CAD build for the part. Positions are in the model's coordinates, mm. A direction names the side the tool comes from. Round coordinates to 2 decimals unless told otherwise and drop trailing zeros. Write each loop counter-clockwise with the first axis right and the second up, starting at its lowest first coordinate (ties: lowest second). Pieces come first, ordered by that corner, then holes. Notation, with made-up numbers: (-15.75, -30) - (37.25, -30) arc R33 cw to (37.25, -2) - close; hole circle Ø6 at (84.5, 77). An arc over 180 degrees is marked (long way). Answer in a Markdown table with one row per item.
```python
from build123d import *

# Parameters (mm, degrees)
F4_DEPTH  = 25.4
F5_DEPTH  = 50.8
F0_R      = 25.4
F0_R_2    = 12.7
F6_DEPTH  = 76.2
F7_DEPTH  = 76.2
F1_W      = 12.7
F1_H      = 34.925
F8_DEPTH  = 25.4
F9_W      = 12.7
F9_H      = 15.875
F10_DEPTH = 25.4


with BuildPart() as f4:
    # F2 (on Front) → F4 (new body, symmetric)
    with BuildSketch(Plane.XZ):
        Polygon((0, 50.8), (0, 0), (38.1, 0), align=None)
    extrude(amount=F4_DEPTH, both=True)

    # F3 (on Right) → F5 (cut)
    with BuildSketch(Plane.YZ):
        with BuildLine():
            ThreePointArc((-25.4, 0), (-21.997045, 12.7), (-12.7, 21.997045))
            Line((-12.7, 21.997045), (-12.7, 38.1))
            Line((-12.7, 38.1), (12.7, 38.1))
            Line((12.7, 38.1), (12.7, 50.8))
            Line((12.7, 50.8), (-25.4, 50.8))
            Line((-25.4, 50.8), (-25.4, 0))
        make_face()
    extrude(amount=F5_DEPTH, mode=Mode.SUBTRACT)

    # F0 (on Right) → F6 (join)
    with BuildSketch(Plane.YZ):
        Circle(F0_R)
        Circle(F0_R_2, mode=Mode.SUBTRACT)
    extrude(amount=F6_DEPTH)

    # F0 (on Right) → F7 (cut)
    with BuildSketch(Plane.YZ):
        Circle(F0_R_2)
    extrude(amount=F7_DEPTH, mode=Mode.SUBTRACT)

    # F1 (on Front) → F8 (cut, symmetric)
    with BuildSketch(Plane.XZ):
        with Locations((57.15, 7.9375)):
            Rectangle(F1_W, F1_H)
    extrude(amount=F8_DEPTH, both=True, mode=Mode.SUBTRACT)

    # F9 (on Front) → F10 (cut, symmetric)
    with BuildSketch(Plane.XZ):
        with Locations((69.85, 17.4625)):
            Rectangle(F9_W, F9_H)
    extrude(amount=F10_DEPTH, both=True, mode=Mode.SUBTRACT)


solid = f4.part
```
Q1. Flat gauge pins, fed straight in: pin 1 (4 mm diameter, centred on x = 58.5, y = -14, fed in from +Z) (3 decimals); pin 2 (10.5 mm diameter, centred on x = 4.5, z = 46.5, fed in from -Y); pin 3 (1.5 mm diameter, centred on x = 17, y = -12.5, fed in from +Z). Where does each tip first touch, or does it go through?
Computed:
| item | result |
|---|---|
| pin 1 | stops at z = -9.525 |
| pin 2 | stops at y = 12.7 |
| pin 3 | stops at z = 29.13 |
Q2. Saw through at A-A on y = 0. List the corners of the cut face in (x, z) (3 decimals).
Computed:
| item | result |
|---|---|
| outline | (0, -25.4) - (76.2, -25.4) - (76.2, -12.7) - (0, -12.7) - close; (0, 12.7) - (50.8, 12.7) - (50.8, 25.4) - (19.05, 25.4) - (9.525, 38.1) - (0, 38.1) - close |
Q3. Drill centre lines: line 1 (Y direction, x = 26.5, z = 0); line 2 (X direction, y = -19, z = -1). Where is each one in solid material? Low to high.
Computed:
| item | result |
|---|---|
| line 1 | y = -25.4 to -12.7, 12.7 to 25.4 |
| line 2 | x = 0 to 50.8, 63.5 to 76.2 |
Q4. Saw through at D-D on x = 68.5. List the corners of the cut face in (y, z) (3 decimals), then the cut area to 3 significant figures.
Computed:
| item | result |
|---|---|
| outline | (-23.546, 9.525) arc R25.4 ccw (long way) to (23.546, 9.525) - (8.4, 9.525) arc R12.7 cw (long way) to (-8.4, 9.525) - close |
| area | 1,020 mm2 |
Q5. Saw through at C-C on x = 42. List the corners of the cut face in (y, z).
Computed:
| item | result |
|---|---|
| outline | circle Ø50.8 at (0, 0); hole circle Ø25.4 at (0, 0) |
Q6. 3-axis set-ups, long thin cutter, end or side, ignore diameter. For faces 4 (the flat face through (4, 12.7, 43)), 5 (the flat face through (70, -16, 9.525)), 6 (the flat face through (63.5, -19, 0)): which of +Z, -Z, +X, -X, +Y, -Y reach the whole face in a straight line?
Computed:
| item | result |
|---|---|
| face 4 | +Z, +X, -X, -Y |
| face 5 | +Z, +X, +Y, -Y |
| face 6 | +Z, +Y, -Y |
Q7. Pull direction X, two halves, no side cores. Call faces 1 (the flat face through (0, 5, 13)), 2 (the flat face through (5, 0, 38.1)), 3 (the flat face through (50.8, 5, 12)): released by +X, released by -X, zero draft, split by the parting line, or undercut.
Computed:
| item | result |
|---|---|
| face 1 | released by -X |
| face 2 | zero draft |
| face 3 | undercut |
Q8. Saw through at B-B on z = -3. List the corners of the cut face in (x, y), then the cut area to 3 significant figures.
Computed:
| item | result |
|---|---|
| outline | (0, -25.22) - (50.8, -25.22) - (50.8, -12.34) - (0, -12.34) - close; (0, 12.34) - (50.8, 12.34) - (50.8, 25.22) - (0, 25.22) - close; (63.5, -25.22) - (76.2, -25.22) - (76.2, -12.34) - (63.5, -12.34) - close; (63.5, 12.34) - (76.2, 12.34) - (76.2, 25.22) - (63.5, 25.22) - close |
| area | 1,640 mm2 |
